```python
from build123d import *

# Parameters (mm, degrees)
SKETCH1_W           = 41
SKETCH1_H           = 28.5
BOSS_EXTRUDE1_DEPTH = 1.6
SKETCH2_W           = 6
SKETCH2_H           = 28
BOSS_EXTRUDE2_DEPTH = 2.5
SKETCH3_W           = 8
SKETCH3_H           = 8
BOSS_EXTRUDE3_DEPTH = 6
SKETCH4_W           = 10
SKETCH4_H           = 6
BOSS_EXTRUDE4_DEPTH = 3.5
SKETCH5_W           = 8
SKETCH5_H           = 16
BOSS_EXTRUDE5_DEPTH = 1.5


with BuildPart() as part:
    # Sketch1 → Boss-Extrude1 (new body)
    with BuildSketch(Plane.XY.offset(13.1)):
        with Locations((-10, 3.5)):
            Rectangle(SKETCH1_W, SKETCH1_H)
    extrude(amount=BOSS_EXTRUDE1_DEPTH)

    # Sketch2 → Boss-Extrude2 (add)
    with BuildSketch(Plane.XY.offset(10.6)):
        with Locations((-10, 3.5)):
            Rectangle(SKETCH2_W, SKETCH2_H)
    extrude(amount=BOSS_EXTRUDE2_DEPTH)

    # Sketch3 → Boss-Extrude3 (add)
    with BuildSketch(Plane.XY.offset(14.7)):
        with Locations((3, 3.5)):
            Rectangle(SKETCH3_W, SKETCH3_H)
    extrude(amount=BOSS_EXTRUDE3_DEPTH)

    # Sketch4 → Boss-Extrude4 (add)
    with BuildSketch(Plane.XY.offset(14.7)):
        with Locations((-20, 3.5)):
            Rectangle(SKETCH4_W, SKETCH4_H)
    extrude(amount=BOSS_EXTRUDE4_DEPTH)

    # Sketch5 → Boss-Extrude5 (add)
    with BuildSketch(Plane.XY.offset(14.7)):
        with Locations((-8, 3.5)):
            Rectangle(SKETCH5_W, SKETCH5_H)
    extrude(amount=BOSS_EXTRUDE5_DEPTH)


solid = part.part
```
Could you check a few things on this model? Use its own coordinates, in mm. A direction names the side the tool comes from. Give positions to 0.01 mm unless a question says otherwise; leave off trailing zeros. Write each loop counter-clockwise with the first axis right and the second up, starting at its lowest first coordinate (ties: lowest second). Pieces come first, ordered by that corner, then holes. Notation, with made-up numbers: (-2.5, 6) - (41.5, 6) arc R22 ccw to (41.5, 45) - close; hole circle Ø8 at (8.5, -9). An arc over 180 degrees is marked (long way). One line per item, written item: value. Start each with the question number.
Item 1: Please list where these lines run through material, in increasing order: line 1 (X direction, y = 2.75, z = 15.75); line 2 (Z direction, x = -27.5, y = 0.75); line 3 (Y direction, x = 3, z = 19). Write a range as from..to.
Item 2: Imagine slicing it at C-C, the plane y = -4. List the corners of the cut face in (x, z) for me, and give its area (3 significant figures).
Item 3: If we mould it in two halves opening along X, with no side actions, what happens to faces 1 (the face through (-20, 0.5, 16)), 2 (the face through (-25, 3, 16)), 3 (the face through (-1, 3, 18)), 4 (the face through (7, 3, 18))? For each: +X half, -X half, draft (parallel to the pull), parting line (faces both ways), or undercut.
Item 4: Imagine slicing it at A-A, the plane z = 16.75. List the corners of the cut face in (x, y) for me, and give its area (3 significant figures).
Item 5: I'm going to push flat-ended pins straight in: pin 1 (2.5 mm diameter, centred on x = -8.5, y = 6.5, fed in from +Z); pin 2 (1.8 mm diameter, centred on y = 2, z = 17, fed in from -X); pin 3 (1.5 mm diameter, centred on x = -8, y = 14.5, fed in from +Z). Where does each tip first touch, or does it pass through?
Item 6: Imagine slicing it at D-D, the plane x = -8.5. List the corners of the cut face in (y, z) for me, and give its area (3 significant figures).
Item 7: Imagine slicing it at B-B, the plane x = 3.5. List the corners of the cut face in (y, z) for me, and give its area (3 significant figures).
Item 8: Which directions (+Z, -Z, +X, -X, +Y, -Y) give clear straight access to the entire face, cutting with the end or side of a thin tool? Please do faces 5 (the face through (-15, 3, 16)), 6 (the face through (3, 7.5, 18)), 7 (the face through (3, -0.5, 18)), 8 (the face through (-10, -10.5, 12)).
Geometry says:
1. line 1: -25..-15, -12..-4, -1..7
1. line 2: 13.1..14.7
1. line 3: -0.5..7.5
2. outline: (-30.5, 13.1) - (-13, 13.1) - (-13, 10.6) - (-7, 10.6) - (-7, 13.1) - (10.5, 13.1) - (10.5, 14.7) - (-4, 14.7) - (-4, 16.2) - (-12, 16.2) - (-12, 14.7) - (-30.5, 14.7) - close
2. area: 92.6 mm^2
3. face 1: draft
3. face 2: -X half
3. face 3: undercut
3. face 4: +X half
4. outline: (-25, 0.5) - (-15, 0.5) - (-15, 6.5) - (-25, 6.5) - close; (-1, -0.5) - (7, -0.5) - (7, 7.5) - (-1, 7.5) - close
4. area: 124 mm^2
5. pin 1: z = 16.2
5. pin 2: x = -25
5. pin 3: z = 14.7
6. outline: (-10.75, 13.1) - (-10.5, 13.1) - (-10.5, 10.6) - (17.5, 10.6) - (17.5, 13.1) - (17.75, 13.1) - (17.75, 14.7) - (11.5, 14.7) - (11.5, 16.2) - (-4.5, 16.2) - (-4.5, 14.7) - (-10.75, 14.7) - close
6. area: 140 mm^2
7. outline: (-10.75, 13.1) - (17.75, 13.1) - (17.75, 14.7) - (7.5, 14.7) - (7.5, 20.7) - (-0.5, 20.7) - (-0.5, 14.7) - (-10.75, 14.7) - close
7. area: 93.6 mm^2
8. face 5: +Z, +Y, -Y
8. face 6: +Z, +X, +Y
8. face 7: +Z, +X, -Y
8. face 8: -Z, +X, -X, -Y
